The model under review builds one solid part; all positions refer to its coordinate system, in mm. A direction names the side the tool comes from. Give positions to 0.01 mm unless a question says otherwise; leave off trailing zeros. Loops run counter-clockwise (first coordinate to the right, second up) from the corner with the lowest first, then second, coordinate; pieces in that order, holes last. Notation, with made-up numbers: M 70,6 L 79,6 A28 ccw 79,35 Z; hole C 44.25,46 d5. An arc over 180 degrees is marked long. One line per item, written item: value. Start each with the question number.
Q1. For faces 4 (the face through (14, -2.5, 5)), 5 (the face through (5.97, 9.36, 4.52)), 6 (the face through (14, 2.5, 5)), 7 (the face through (16.5, -0.07, 4.99)), 8 (the face through (-14, -2.5, 5)), list the 3-axis set-ups (+Z, -Z, +X, -X, +Y, -Y) from which the entire face can be reached by the end or side of a thin tool; tool diameter is ignored.
Q2. We need section A-A on y = 0. Write out the cut boundary in (x, z).
Q3. Mouldability with a two-part tool opening along Y and no side actions: class faces 1 (the face through (13.7, -1.1, 4)), 2 (the face through (-14, 2.5, 5)), 3 (the face through (-16.5, 0.07, 4.99)) as released by +Y, released by -Y, zero draft, split by the parting line, or undercut.
Q4. For pin 1 (1.6 mm diameter, centred on x = 13.5, z = 4.5, fed in from -Y); pin 2 (2 mm diameter, centred on x = 5, y = 0.5, fed in from +Z); pin 3 (9 mm diameter, centred on x = 0, y = 0, fed in from +Z); pin 4 (1 mm diameter, centred on x = 14, z = 5, fed in from +Y), all flat-tipped, find the tip position at first contact; note any pin that passes through.
Q5. We need section C-C on z = 5.6. Write out the cut boundary in (x, y), plus the area to 3 significant figures.
Q6. To check wall thickness, follow line 1 along Y through (x, z) = (15, 5.45); line 2 along X through (y, z) = (0, 2.15); line 3 along X through (y, z) = (5, 3.1). State the ranges of each line that lie inside material, in increasing order. Write a range as from..to.
Q7. We need section B-B on x = 0. Write out the cut boundary in (y, z), plus the area to 3 significant figures.
Q8. We need section D-D on y = -3.5. Write out the cut boundary in (x, z).
```python
from build123d import *

# Parameters (mm, degrees)
SKETCH2_R           = 12.5
SKETCH2_R_2         = 5
BOSS_EXTRUDE3_DEPTH = 6
SKETCH4_R           = 11.1
CUT_EXTRUDE1_DEPTH  = 3
BOSS_EXTRUDE4_START = -2
SKETCH5_R           = 1.5
BOSS_EXTRUDE4_DEPTH = 2


with BuildPart() as part:
    # Sketch2 → Boss-Extrude3 (new body)
    with BuildSketch(Plane.XY):
        Circle(SKETCH2_R)
        Circle(SKETCH2_R_2, mode=Mode.SUBTRACT)
    extrude(amount=BOSS_EXTRUDE3_DEPTH)

    # Sketch4 → Cut-Extrude1 (cut)
    with BuildSketch(Plane.XY.offset(6)):
        Circle(SKETCH4_R)
    extrude(amount=-CUT_EXTRUDE1_DEPTH, mode=Mode.SUBTRACT)

    # Sketch5 → Boss-Extrude4 (add)
    # profile 1 of 2: a face of its own
    with BuildSketch(Plane.XY.offset(6).offset(BOSS_EXTRUDE4_START)):
        with BuildLine():
            Line((-15, 2.5), (-12.247448714, 2.5))
            ThreePointArc((-12.247448714, 2.5), (-12.5, 0), (-12.247448714, -2.5))
            Line((-12.247448714, -2.5), (-15, -2.5))
            ThreePointArc((-15, -2.5), (-17.5, 0), (-15, 2.5))
        make_face()
        with Locations((-15, 0)):
            Circle(SKETCH5_R, mode=Mode.SUBTRACT)
    # profile 2 of 2: a face of its own
    with BuildSketch(Plane.XY.offset(6).offset(BOSS_EXTRUDE4_START)):
        with BuildLine():
            Line((15, -2.5), (12.247448714, -2.5))
            ThreePointArc((12.247448714, -2.5), (12.5, 0), (12.247448714, 2.5))
            Line((12.247448714, 2.5), (15, 2.5))
            ThreePointArc((15, 2.5), (17.5, 0), (15, -2.5))
        make_face()
        with Locations(Location((15, 0, 0), (0, 0, 180))):
            Circle(SKETCH5_R, mode=Mode.SUBTRACT)
    extrude(amount=BOSS_EXTRUDE4_DEPTH)


solid = part.part
```
Solved:
1. face 4: +Z, -Z, +X, -Y
1. face 5: +Z
1. face 6: +Z, -Z, +X, +Y
1. face 7: +Z, -Z
1. face 8: +Z, -Z, -X, -Y
2. outline: M -17.5,4 L -16.5,4 L -16.5,6 L -17.5,6 Z; M -13.5,4 L -12.5,4 L -12.5,0 L -5,0 L -5,3 L -11.1,3 L -11.1,6 L -13.5,6 Z; M 5,0 L 12.5,0 L 12.5,4 L 13.5,4 L 13.5,6 L 11.1,6 L 11.1,3 L 5,3 Z; M 16.5,4 L 17.5,4 L 17.5,6 L 16.5,6 Z
3. face 1: zero draft
3. face 2: released by +Y
3. face 3: undercut
4. pin 1: y = -2.5
4. pin 2: z = 3
4. pin 3: through
4. pin 4: y = 2.5
5. outline: M -15,-2.5 L -12.25,-2.5 A12.5 ccw 12.25,-2.5 L 15,-2.5 A2.5 ccw 15,2.5 L 12.25,2.5 A12.5 ccw -12.25,2.5 L -15,2.5 A2.5 ccw Z; hole C -15,0 d3; hole C 0,0 d22.2; hole C 15,0 d3
5. area: 135 mm2
6. line 1: -2.5..-1.5, 1.5..2.5
6. line 2: -12.5..-5, 5..12.5
6. line 3: -11.46..-9.91, 9.91..11.46
7. outline: M -12.5,0 L -5,0 L -5,3 L -11.1,3 L -11.1,6 L -12.5,6 Z; M 5,0 L 12.5,0 L 12.5,6 L 11.1,6 L 11.1,3 L 5,3 Z
7. area: 53.4 mm2
8. outline: M -12,0 L -3.57,0 L -3.57,3 L -10.53,3 L -10.53,6 L -12,6 Z; M 3.57,0 L 12,0 L 12,6 L 10.53,6 L 10.53,3 L 3.57,3 Z
